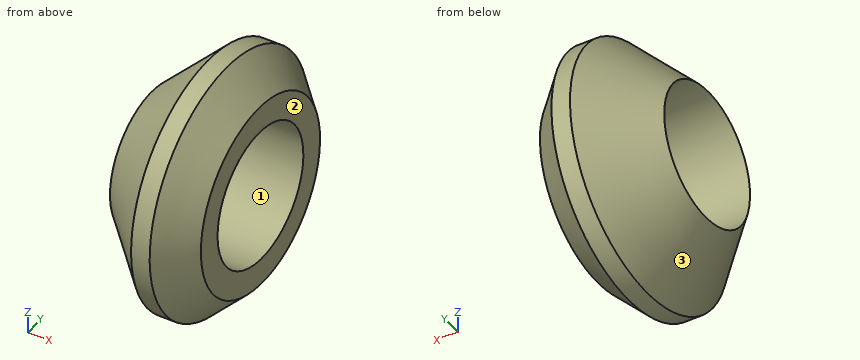
Autodesk Inventor part; units mm, degrees
ref_plane "YZ Plane" through (0, 0, 0) normal (1, 0, 0) x (0, 1, 0)
ref_plane "XZ Plane" through (0, 0, 0) normal (0, 1, 0) x (-1, 0, 0)
ref_plane "XY Plane" through (0, 0, 0) normal (0, 0, 1) x (1, 0, 0)
sketch "Sketch1" plane through (0, 0, 0) normal (0, 1, 0) x (-1, 0, 0)
  line L0 (0, 0) -> (5.4483, 0)
  line L1 (5.4483, 0) -> (5.4483, -3.429) construction
  line L2 (5.4483, -3.429) -> (0, -3.429)
  line L3 (0, -3.429) -> (0, 0) construction
  line L4 (5.4483, -3.429) -> (0, -3.429)
  line L5 (0, -3.429) -> (0, -6.35)
  line L6 (0, -6.35) -> (5.4483, -6.35)
  line L7 (5.4483, -6.35) -> (5.4483, -3.429)
  dimension "d0" = 5.4483
  dimension "d1" = 3.429
  dimension "d2" = 6.35
revolve "Revolution1" add sketch "Sketch1" angle 360 about axis through (0, 0, 0) along (-1, 0, 0)
chamfer "Chamfer1" distance 2.921 angle 45 1 edges at (-5.4483, 0, 6.35)
chamfer "Chamfer2" distance 1.5875 angle 45 1 edges at (0, 0, 6.35)
properties part number "Spacer" material "Nylon 6/6"
Geometry: final body of the model. Coordinates: model frame, mm. Face numbers are marked on the shaded views. Round coordinates to 2 decimals unless told otherwise and drop trailing zeros. Order: outer loops, then holes, each group sorted by start corner. A loop starts at its lowest first (then second) coordinate and runs counter-clockwise, first axis right, second up. Notation, with made-up numbers: M -18,-7 L 29,-7 A15 cw 29,9 Z; hole C 21.5,39 d2. An arc over 180 degrees is marked long. Use one line per item in the form item = value. Start each with the question number.
Q1. Material intervals for line 1 (Z direction, x = -2.45, y = 0); line 2 (Z direction, x = -0.6, y = 0.25); line 3 (Y direction, x = -4.75, z = -2.5), sorted ascending. Write a range as [from, to].
Q2. Cut plane C-C (x = -2.95). Return loops of the section in (y, z).
Q3. Mould query, pull axis Z, two halves, no side actions, for the marked faces 1, 2 and 3. Classes: +Z half, -Z half, draft (parallel to the pull), parting line (faces both ways), or undercut.
Q4. Cut plane D-D (x = -0.5). Return loops of the section in (y, z) (1 decimal).
Q5. Pin query (flat end, axial travel): pin 1 Ø3 at (y, z) = (-4, -5) entering from +X; pin 2 Ø1.5 at (x, y) = (-4, 2) entering from +Z; pin 3 Ø1 at (x, z) = (-2, 4) entering from -Y; pin 4 Ø3 at (y, z) = (-2.5, 1.5) entering from -X. Return the tip coordinate at first contact, or that it passes through.
Geometry results:
q1.line_1 = [-6.35, -3.43], [3.43, 6.35]
q1.line_2 = [-5.36, -3.42], [3.42, 5.36]
q1.line_3 = [-3.28, -2.35], [2.35, 3.28]
q2.outline = C 0,0 d11.86; hole C 0,0 d6.86
q3.face_1 = undercut
q3.face_2 = draft
q3.face_3 = parting line
q4.outline = C 0,0 d10.5; hole C 0,0 d6.9
q5.pin_1 = -0.14
q5.pin_2 = 5.3
q5.pin_3 = -5.3
q5.pin_4 = -5.45
